Autodesk Inventor part; units mm, degrees
ref_plane "YZ Plane" through (0, 0, 0) normal (1, 0, 0) x (0, 1, 0)
ref_plane "XZ Plane" through (0, 0, 0) normal (0, 1, 0) x (-1, 0, 0)
ref_plane "XY Plane" through (0, 0, 0) normal (0, 0, 1) x (1, 0, 0)
sketch "スケッチ1" plane through (0, 0, 0) normal (0, 0, 1) x (1, 0, 0)
  line L0 (0, 0) -> (-94.2, 0)
  line L1 (-94.2, 0) -> (-94.2, -12)
  line L2 (-94.2, -12) -> (0, -12)
  line L3 (0, -12) -> (0, 0)
  circle A0 centre (-85.5, -2) radius 1.1
  circle A1 centre (-85.5, -10) radius 1.1
  circle A2 centre (-35.5, -10) radius 1.1
  circle A3 centre (-35.5, -2) radius 1.1
  dimension "d0" = 94.2
  dimension "d1" = 12
  dimension "d2" = 2.2
  dimension "d3" = 2.2
  dimension "d4" = 8.7
  dimension "d5" = 2.2
  dimension "d7" = 2.2
  dimension "d9" = 50
  dimension "d10" = 50
extrude "押し出し1" add sketch "スケッチ1" along normal blind 1.5
sketch "スケッチ2" plane through (0, 0, 1.5) normal (0, 0, 1) x (1, 0, 0)
  line L0 (0, 2.5) -> (0, -14.5)
  line L1 (0, -14.5) -> (-20, -14.5)
  line L2 (-20, -14.5) -> (-22.5, -12)
  line L3 (-94.2, -12) -> (0, -12)
  line L4 (-22.5, -12) -> (-22.5, 0)
  line L5 (0, 0) -> (-94.2, 0)
  line L6 (0, 2.5) -> (-20, 2.5)
  line L7 (-20, 2.5) -> (-22.5, 0)
  dimension "d17" = 17
  dimension "d18" = 20
  dimension "d19" = 135
extrude "押し出し2" add sketch "スケッチ2" against normal blind 1.5
sketch "スケッチ3" plane through (0, 0, 1.5) normal (0, 0, 1) x (1, 0, 0)
  circle A0 centre (-5.5, -12) radius 1.1
  circle A1 centre (-5.5, 0) radius 1.1
  point P0 (0, 0)
  dimension "d22" = 2.2
  dimension "d23" = 2.2
extrude "押し出し3" cut sketch "スケッチ3" against normal blind 1.5
sketch "スケッチ4" plane through (0, 0, 1.5) normal (0, 0, 1) x (1, 0, 0)
  line L0 (0, -14.5) -> (0, 2.5)
  line L1 (0, -6) -> (14, -6)
  line L2 (0, -6) -> (14, -6) construction
  line L3 (-20, -14.5) -> (0, -14.5)
  line L4 (0, -14.5) -> (14, -14.5)
  line L5 (14, -14.5) -> (14, 2.5)
  line L6 (-20, 2.5) -> (0, 2.5)
  line L7 (14, 2.5) -> (0, 2.5)
  line L8 (0, 2.5) -> (0, -14.5)
  circle A0 centre (7, -12) radius 1.1
  circle A1 centre (7, 0) radius 1.1
  point P0 (0, 0)
  dimension "d27" = 14
  dimension "d28" = 0
  dimension "d29" = 2.2
  dimension "d30" = 2.2
extrude "押し出し4" add sketch "スケッチ4" against normal blind 1.5
fillet "フィレット3" radius 0.5 8 edges at (14, 2.5, 0.75) (-20, 2.5, 0.75) (-22.5, 0, 0.75) (-94.2, 0, 0.75) (-94.2, -12, 0.75) (-22.5, -12, 0.75) (-20, -14.5, 0.75) (14, -14.5, 0.75)
properties part number "slider_plate" material "アルミニウム"
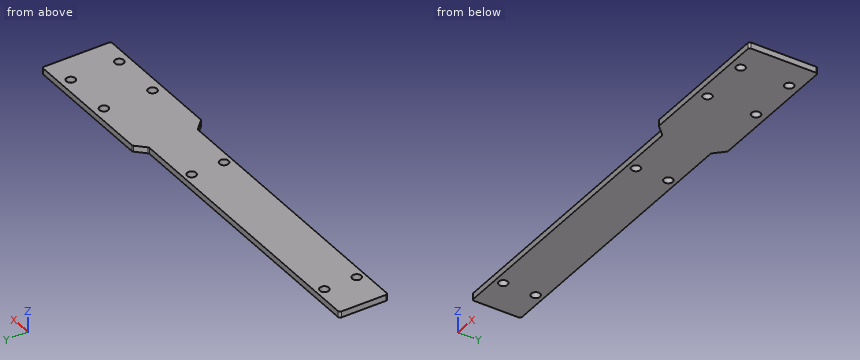
Build history of the part. All positions in model axes, mm. Round coordinates to 2 decimals unless told otherwise and drop trailing zeros. Write each loop counter-clockwise with the first axis right and the second up, starting at its lowest first coordinate (ties: lowest second). Pieces come first, ordered by that corner, then holes. Notation, with made-up numbers: (17, 75.25) - (52, 75.25) arc R20 cw to (52, 85.25) - close; hole circle Ø7 at (83.25, 81). An arc over 180 degrees is marked (long way). Answer as CSV lines item,"result".
Q1. Cut at C-C (y = -10). Write the cut outline in (x, z).
Report:
outline,"(-94.2, 0) - (-86.6, 0) - (-86.6, 1.5) - (-94.2, 1.5) - close; (-84.4, 0) - (-36.6, 0) - (-36.6, 1.5) - (-84.4, 1.5) - close; (-34.4, 0) - (14, 0) - (14, 1.5) - (-34.4, 1.5) - close"
Q2. Cut at D-D (x = -52). Write the cut outline in (y, z), and give its area (3 significant figures).
Report:
outline,"(-12, 0) - (0, 0) - (0, 1.5) - (-12, 1.5) - close"
area,"18.0 mm^2"
Q3. Cut at A-A (x = -85.5). Write the cut outline in (y, z).
Report:
outline,"(-12, 0) - (-11.1, 0) - (-11.1, 1.5) - (-12, 1.5) - close; (-8.9, 0) - (-3.1, 0) - (-3.1, 1.5) - (-8.9, 1.5) - close; (-0.9, 0) - (0, 0) - (0, 1.5) - (-0.9, 1.5) - close"
Q4. Drop a flat-ended pin along its axis: pin 1 (2.5 mm diameter, centred on x = -35.5, y = -2, fed in from +Z). Give the stop position or say it passes through.
Report:
pin 1,"stops at z = 1.5"
Q5. Cut at B-B (z = 0.9). State how many separate pieces and enclosed holes the cut face has, and give its area (3 significant figures).
Report:
separate pieces,"1"
enclosed holes,"8"
area,"1,440 mm^2"
Q6. Drill centre lines: probe 1 along Y at (x, z) = (-85.5, 1.2); probe 2 along X at (y, z) = (1, 0.95); probe 3 along X at (y, z) = (-11.5, 0.45). Where is each one in solid material? Low to high. Write a range as [from, to].
Report:
probe 1,"y = [-12, -11.1], [-8.9, -3.1], [-0.9, 0]"
probe 2,"x = [-21.5, -5.96], [-5.04, 6.54], [7.46, 14]"
probe 3,"x = [-94.2, -6.48], [-4.52, 6.02], [7.98, 14]"
